Geometry check sheet. Reference: the model listing, model coordinates, mm. Round coordinates to 2 decimals unless told otherwise and drop trailing zeros. Write each loop counter-clockwise with the first axis right and the second up, starting at its lowest first coordinate (ties: lowest second). Pieces come first, ordered by that corner, then holes. Notation, with made-up numbers: M -28,-4.75 L 7,-4.75 A28 cw 7,27.25 Z; hole C -7,-22.75 d7. An arc over 180 degrees is marked long. Answer as CSV lines item,"result". Start each with the question number.
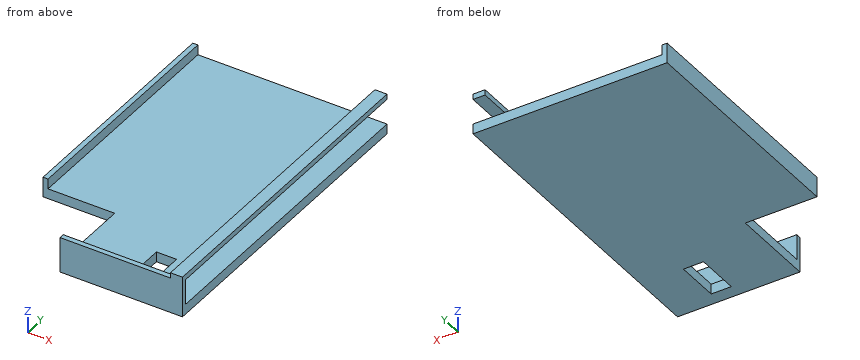
```python
from build123d import *

# Parameters (mm, degrees)
F0_W     = 6.35
F0_H     = 13.716
F1_DEPTH = 3.175
F0_W_2   = 1.5875
F0_H_2   = 73.952875
F2_DEPTH = 6.35
F0_W_3   = 38.6812536
F0_H_3   = 1.5875
F3_DEPTH = 11.176
F7_DEPTH = 3.81


# Not quite as in the source:
# - a feature names something its author has since deleted; it is built from what else it names


with BuildPart() as f1:
    # F0 (on Top) → F1 (new body)
    with BuildSketch(Plane.XY):
        Polygon((29.8689268, -49.6764375), (29.8689268, 49.6764375), (-29.8689268, 49.6764375), (-29.8689268, -24.2764375), (-8.8123268, -24.2764375), (-8.8123268, -49.6764375), align=None)
        with Locations((13.4126732, -40.2784375)):
            Rectangle(F0_W, F0_H, mode=Mode.SUBTRACT)
    extrude(amount=F1_DEPTH)

    # F0 (on Top) → F2 (join)
    with BuildSketch(Plane.XY):
        with Locations((-30.6626768, 12.7)):
            Rectangle(F0_W_2, F0_H_2)
    extrude(amount=F2_DEPTH)

    # F0 (on Top) → F3 (join)
    with BuildSketch(Plane.XY):
        with Locations((10.5283, -50.4701875)):
            Rectangle(F0_W_3, F0_H_3)
    extrude(amount=F3_DEPTH)

    # F6 (on face) → F7 (join)
    with BuildSketch(Plane.YZ.offset(29.8689268)):
        Polygon((-51.2639375, 12.8905), (-51.2639375, 11.176), (-49.6764375, 11.176), (49.6764375, 11.176), (49.6764375, 12.8905), align=None)
    extrude(amount=-F7_DEPTH)


solid = f1.part
```
1) Section check C-C, the plane y = -38. Record the cut outline in (x, z) (1 decimal).
2) Scan lines: line 1 (Z direction, x = 26.5, y = -44) (1 decimal); line 2 (Z direction, x = 6, y = 12) (3 decimals); line 3 (Y direction, x = 3.5, z = 5). Record each from-to range of solid material in increasing order. Write a range as from..to.
3) Section check D-D, the plane x = 21. Record the cut outline in (y, z) (3 decimals).
4) Section check B-B, the plane z = 1.25. Record the cut outline in (x, y).
5) Go/stop test with flat-tipped pins: pin 1 (3.5 mm diameter, centred on y = 12, z = 5.5, fed in from +X); pin 2 (3.5 mm diameter, centred on y = -42, z = 1, fed in from -X); pin 3 (1.3 mm diameter, centred on x = -31, y = -5.5, fed in from +Z). Record where each tip stops, or that it passes through.
Results:
1,outline,"M -8.8,0 L 10.2,0 L 10.2,3.2 L -8.8,3.2 Z; M 16.6,0 L 29.9,0 L 29.9,3.2 L 16.6,3.2 Z; M 26.1,11.2 L 29.9,11.2 L 29.9,12.9 L 26.1,12.9 Z"
2,line 1,"z = 0..3.2, 11.2..12.9"
2,line 2,"z = 0..3.175"
2,line 3,"y = -51.26..-49.68"
3,outline,"M -51.264,0 L 49.676,0 L 49.676,3.175 L -49.676,3.175 L -49.676,11.176 L -51.264,11.176 Z"
4,outline,"M -31.46,-24.28 L -8.81,-24.28 L -8.81,-51.26 L 29.87,-51.26 L 29.87,49.68 L -31.46,49.68 Z; hole M 10.24,-47.14 L 16.59,-47.14 L 16.59,-33.42 L 10.24,-33.42 Z"
5,pin 1,"stops at x = -29.87"
5,pin 2,"stops at x = -8.81"
5,pin 3,"stops at z = 6.35"
